```python
from build123d import *

# Parameters (mm, degrees)
SKETCH1_R               = 20
SKETCH1_R_2             = 16.01
BOSS_EXTRUDE1_DEPTH     = 70
CUT_EXTRUDE1_DEPTH      = 76.498344353
CUT_EXTRUDE1_DEPTH_BACK = 76.498344353
SKETCH3_R               = 16.01
BOSS_EXTRUDE2_DEPTH     = 30
CUT_EXTRUDE2_DEPTH      = 49.590122453
CUT_EXTRUDE2_DEPTH_BACK = 49.590122453
SKETCH4_R               = 3.326


with BuildPart() as part:
    # Sketch1 → Boss-Extrude1 (new body)
    with BuildSketch(Plane(origin=(0, 0, 0), x_dir=(1, 0, 0), z_dir=(0, 1, 0))):
        with Locations(Location((0, 0, 0), (0, 0, 270))):
            Circle(SKETCH1_R)
        with Locations(Location((0, 0, 0), (0, 0, 270))):
            Circle(SKETCH1_R_2, mode=Mode.SUBTRACT)
    extrude(amount=BOSS_EXTRUDE1_DEPTH)

    # Sketch2 → Cut-Extrude1 (cut, two sides: drawn at the far end of the back side and taken through both)
    with BuildSketch(Plane(origin=(0, 70, 0), x_dir=(1, 0, 0), z_dir=(0, 1, 0)).offset(-CUT_EXTRUDE1_DEPTH_BACK)):
        with BuildLine():
            Line((-19, -6.244997998), (-19, 6.244997998))
            ThreePointArc((-19, 6.244997998), (-20, 0), (-19, -6.244997998))
        make_face()
        with BuildLine():
            Line((-5.4292033, -19.24899352), (-19, -6.244997998))
            ThreePointArc((-19, -6.244997998), (-13.837357709, -14.44048239), (-5.4292033, -19.24899352))
        make_face()
        with BuildLine():
            ThreePointArc((5.4292033, -19.24899352), (13.837357709, -14.44048239), (19, -6.244997998))
            Line((19, -6.244997998), (5.4292033, -19.24899352))
        make_face()
        with BuildLine():
            Line((0, -19.24899352), (-5.4292033, -19.24899352))
            ThreePointArc((-5.4292033, -19.24899352), (-2.740449745, -19.811358742), (0, -20))
            Line((0, -20), (0, -19.24899352))
        make_face()
        with BuildLine():
            Line((5.4292033, -19.24899352), (0, -19.24899352))
            Line((0, -19.24899352), (0, -20))
            ThreePointArc((0, -20), (2.740449745, -19.811358742), (5.4292033, -19.24899352))
        make_face()
        with BuildLine():
            ThreePointArc((20, 0), (19.748417658, 3.16227766), (19, 6.244997998))
            Line((19, 6.244997998), (19, -6.244997998))
            ThreePointArc((19, -6.244997998), (19.748417658, -3.16227766), (20, 0))
        make_face()
    extrude(amount=CUT_EXTRUDE1_DEPTH + CUT_EXTRUDE1_DEPTH_BACK, mode=Mode.SUBTRACT)

    # Sketch3 → Boss-Extrude2 (add)
    with BuildSketch(Plane.XZ):
        with Locations(Location((0, 0, 0), (0, 0, 270))):
            Circle(SKETCH3_R)
    extrude(amount=-BOSS_EXTRUDE2_DEPTH)

    # Sketch4 → Cut-Extrude2 (cut, two sides: drawn at the far end of the back side and taken through both)
    with BuildSketch(Plane(origin=(0, 30, 0), x_dir=(1, 0, 0), z_dir=(0, 1, 0)).offset(-CUT_EXTRUDE2_DEPTH_BACK)):
        with Locations(Location((0, 0, 0), (0, 0, 270))):
            Circle(SKETCH4_R)
    extrude(amount=CUT_EXTRUDE2_DEPTH + CUT_EXTRUDE2_DEPTH_BACK, mode=Mode.SUBTRACT)


solid = part.part
```
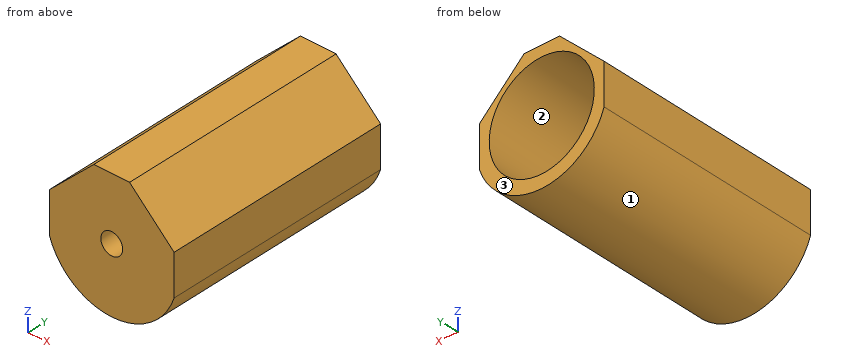
Geometry check sheet. Reference: the model listing, model coordinates, mm. Face numbers are marked on the shaded views. Round coordinates to 2 decimals unless told otherwise and drop trailing zeros. Loops run counter-clockwise (first coordinate to the right, second up) from the corner with the lowest first, then second, coordinate; pieces in that order, holes last. Notation, with made-up numbers: (22, 51) - (52, 51) arc R34 cw to (52, 89) - close; hole circle Ø7 at (-29, 24). An arc over 180 degrees is marked (long way). Use a Markdown table: item, result.
Q1. Cross-section at D-D on z = -12.5. Record the cut outline in (x, y).
Solutions:
| item | result |
|---|---|
| outline | (-15.61, 0) - (15.61, 0) - (15.61, 70) - (10, 70) - (10, 30) - (-10, 30) - (-10, 70) - (-15.61, 70) - close |
Q2. Draft check along Z on the marked faces 1, 2 and 3. Enter one of: released by +Z, released by -Z, zero draft, split by the parting line, or undercut.
Solutions:
| item | result |
|---|---|
| face 1 | released by -Z |
| face 2 | undercut |
| face 3 | zero draft |
Q3. Cross-section at B-B on y = 16.5. Record the cut outline in (x, z) (3 decimals), plus the area to 3 significant figures.
Solutions:
| item | result |
|---|---|
| outline | (-19, -6.245) arc R20 ccw to (19, -6.245) - (19, 6.245) - (5.429, 19.249) - (-5.429, 19.249) - (-19, 6.245) - close; hole circle Ø6.652 at (0, 0) |
| area | 1,140 mm2 |
Q4. Cross-section at A-A on z = 0. Record the cut outline in (x, y).
Solutions:
| item | result |
|---|---|
| outline | (-19, 0) - (-3.33, 0) - (-3.33, 30) - (-16.01, 30) - (-16.01, 70) - (-19, 70) - close; (3.33, 0) - (19, 0) - (19, 70) - (16.01, 70) - (16.01, 30) - (3.33, 30) - close |
Q5. Go/stop test with flat-tipped pins: P1, Ø12, axis at x = 8.5, z = -14.5, coming from the -Y side; P2, Ø5, axis at x = -8.5, y = 52.5, coming from the -Z side; P3, Ø4, axis at x = 3.5, y = 10.5, coming from the -Z side; P4, Ø4, axis at x = 9, y = 50, coming from the -Z side (3 decimals). Record where each tip stops, or that it passes through.
Solutions:
| item | result |
|---|---|
| P1 | stops at y = 0 |
| P2 | stops at z = -19.08 |
| P3 | stops at z = -19.94 |
| P4 | stops at z = -18.735 |
Q6. Material ranges on line 1 (Z direction, x = 0, y = 48); line 2 (Z direction, x = 0, y = 15); line 3 (X direction, y = 22.75, z = 0), recorded low to high.
Solutions:
| item | result |
|---|---|
| line 1 | z = -20 to -16.01, 16.01 to 19.25 |
| line 2 | z = -20 to -3.33, 3.33 to 19.25 |
| line 3 | x = -19 to -3.33, 3.33 to 19 |
Q7. Cross-section at C-C on x = -12. Record the cut outline in (y, z), plus the area to 3 significant figures.
Solutions:
| item | result |
|---|---|
| outline | (0, -16) - (70, -16) - (70, -10.6) - (30, -10.6) - (30, 10.6) - (70, 10.6) - (70, 12.95) - (0, 12.95) - close |
| area | 1,180 mm2 |
